from build123d import *

# Parameters (mm, degrees)
BOSS_EXTRUDE1_DEPTH = 35
SKETCH2_R           = 1.6
CUT_EXTRUDE1_DEPTH  = 51.655700568
CUT_EXTRUDE2_START  = -3
CUT_EXTRUDE2_DEPTH  = 48.655700568
FILLET1_R           = 5


with BuildPart() as part:
    # Sketch1 → Boss-Extrude1 (new body)
    with BuildSketch(Plane.XY):
        Polygon((0, 0), (21, 30), (21, 0), align=None)
    extrude(amount=BOSS_EXTRUDE1_DEPTH)

    # Sketch2 → Cut-Extrude1 (cut, through all)
    with BuildSketch(Plane.XZ):
        with Locations((10, 27.5)):
            Circle(SKETCH2_R)
        with Locations(Location((10, 7.5, 0), (0, 0, 180))):
            Circle(SKETCH2_R)
    extrude(amount=-CUT_EXTRUDE1_DEPTH, mode=Mode.SUBTRACT)

    # Sketch3 → Cut-Extrude2 (cut, through all)
    with BuildSketch(Plane.XZ.offset(CUT_EXTRUDE2_START)):
        Polygon((13.233161507, 27.5), (11.616580754, 30.3), (8.383419246, 30.3), (6.766838493, 27.5), (8.383419246, 24.7), (11.616580754, 24.7), align=None)
        Polygon((13.233161507, 7.5), (11.616580754, 10.3), (8.383419246, 10.3), (6.766838493, 7.5), (8.383419246, 4.7), (11.616580754, 4.7), align=None)
    extrude(amount=-CUT_EXTRUDE2_DEPTH, mode=Mode.SUBTRACT)

    # Fillet1
    # the kernel refuses this fillet: 5 mm, written as the material it takes off along each edge
    with BuildSketch(Plane(origin=(21, 30, -39.6545636), x_dir=(-0.5734623443633282, -0.8192319205190405, 0), z_dir=(0, 0, 1))) as fillet1_piece_1:
        with BuildLine():
            CenterArc((FILLET1_R * 3.17236508796, FILLET1_R), FILLET1_R, 124.992020199, 145.007979801)
            Line((FILLET1_R * 2.5989027436, FILLET1_R * 1.81923192052), (0, 0))
            Line((0, 0), (FILLET1_R * 3.17236508796, 0))
        make_face()
    extrude(amount=114.309127199, mode=Mode.SUBTRACT)


solid = part.part
The listing builds one solid part. Answer for the finished solid, in the listing's coordinates (mm). A direction names the side the tool comes from. Give positions to 0.01 mm unless a question says otherwise; leave off trailing zeros. Loops run counter-clockwise (first coordinate to the right, second up) from the corner with the lowest first, then second, coordinate; pieces in that order, holes last.
Item 1: A cutting plane is placed at C-C (y = 13.75). Give the vertices of the cut face in (x, z) (3 decimals), then the cut area to 3 significant figures.
Derived:
outline: (9.625, 0) - (21, 0) - (21, 35) - (9.625, 35) - (9.625, 30.3) - (11.617, 30.3) - (13.233, 27.5) - (11.617, 24.7) - (9.625, 24.7) - (9.625, 10.3) - (11.617, 10.3) - (13.233, 7.5) - (11.617, 4.7) - (9.625, 4.7) - close
area: 367 mm2
Item 2: A cutting plane is placed at D-D (z = 20.5). Give the vertices of the cut face in (x, y).
Derived:
outline: (0, 0) - (21, 0) - (21, 14.14) arc R5 ccw to (11.9, 17.01) - close
Item 3: A cutting plane is placed at A-A (y = 5). Give the vertices of the cut face in (x, z), then the cut area to 3 significant figures.
Derived:
outline: (3.5, 0) - (21, 0) - (21, 35) - (3.5, 35) - close; hole (6.77, 7.5) - (8.38, 4.7) - (11.62, 4.7) - (13.23, 7.5) - (11.62, 10.3) - (8.38, 10.3) - close; hole (6.77, 27.5) - (8.38, 24.7) - (11.62, 24.7) - (13.23, 27.5) - (11.62, 30.3) - (8.38, 30.3) - close
area: 558 mm2
Item 4: A tool of negligible diameter and unlimited length cuts with its end or side. For faces 1 (the flat face through (7.564, 6.428, 26.12)), 2 (the cylindrical face through (8.82, 1.48, 28.58)), from which of +Z, -Z, +X, -X, +Y, -Y can it reach the whole face along a straight path? Write none if from no direction.
Derived:
face 1: +Y
face 2: +Y, -Y
Item 5: Each of these flat-tipped pins is pushed along its axis until it touches: pin 1 Ø1.9 at (x, z) = (10, 27.5) entering from +Y; pin 2 Ø6 at (x, z) = (10.5, 13) entering from +Y; pin 3 Ø5 at (x, z) = (10, 7.5) entering from +Y. Where does it stop, or does it pass through?
Derived:
pin 1: passes through
pin 2: stops at y = 18.47
pin 3: stops at y = 3
Item 6: Determine the mould class of faces 3 (the flat face through (13, 8, 0)), 4 (the flat face through (21, 7, 17)), 5 (the flat face through (12.414, 10.544, 26.08)) for opening direction Z: +Z half, -Z half, draft (parallel to the pull), parting line (faces both ways), or undercut.
Derived:
face 3: -Z half
face 4: draft
face 5: undercut
Item 7: Find the intervals of material crossed by line 1 along Z through (x, y) = (10, 1.45); line 2 along X through (y, z) = (0.85, 7.5) (3 decimals); line 3 along X through (y, z) = (4.5, 30), in increasing order.
Derived:
line 1: z = 0 to 5.9, 9.1 to 25.9, 29.1 to 35
line 2: x = 0.595 to 8.4, 11.6 to 21
line 3: x = 3.15 to 8.21, 11.79 to 21
Item 8: A cutting plane is placed at B-B (x = 10). Give the vertices of the cut face in (y, z), then the cut area to 3 significant figures.
Derived:
outline: (0, 0) - (14.29, 0) - (14.29, 4.7) - (3, 4.7) - (3, 5.9) - (0, 5.9) - close; (0, 9.1) - (3, 9.1) - (3, 10.3) - (14.29, 10.3) - (14.29, 24.7) - (3, 24.7) - (3, 25.9) - (0, 25.9) - close; (0, 29.1) - (3, 29.1) - (3, 30.3) - (14.29, 30.3) - (14.29, 35) - (0, 35) - close
area: 354 mm2
